```python
from build123d import *

# Parameters (mm, degrees)
F0_R     = 2.1
F1_DEPTH = 4


with BuildPart() as f1:
    # F0 (on Front) → F1 (new body)
    with BuildSketch(Plane.XZ):
        with BuildLine():
            ThreePointArc((-26.381971, 6.326054), (-23.972685, 2.787165), (-22.959026, -1.372268))
            ThreePointArc((-22.959026, -1.372268), (-21.551931, -8.032077), (-18.25719, -13.988388))
            ThreePointArc((-18.25719, -13.988388), (-14.253779, -16.291001), (-9.800476, -15.067308))
            Line((-9.800476, -15.067308), (-7.628003, -13.369986))
            ThreePointArc((-7.628003, -13.369986), (-5.887443, -12.424939), (-3.934034, -12.098051))
            Line((-3.934034, -12.098051), (3.934034, -12.098051))
            ThreePointArc((3.934034, -12.098051), (5.887443, -12.424939), (7.628003, -13.369986))
            Line((7.628003, -13.369986), (9.800476, -15.067308))
            ThreePointArc((9.800476, -15.067308), (14.253779, -16.291001), (18.25719, -13.988388))
            ThreePointArc((18.25719, -13.988388), (18.941172, 13.047299), (-6.562939, 22.043771))
            ThreePointArc((-6.562939, 22.043771), (-10.818219, 21.573689), (-14.967711, 22.627305))
            Line((-14.967711, 22.627305), (-29.819204, 29.402617))
            ThreePointArc((-29.819204, 29.402617), (-38.582061, 27.01545), (-37.828191, 17.964599))
            Line((-37.828191, 17.964599), (-26.381971, 6.326054))
        make_face()
        with BuildLine():
            ThreePointArc((11.244166, -10.473286), (9.304982, -9.523645), (7.182465, -9.127198))
            ThreePointArc((7.182465, -9.127198), (6.591412, -9.105339), (6, -9.098051))
            Line((6, -9.098051), (-6, -9.098051))
            ThreePointArc((-6, -9.098051), (-6.591412, -9.105339), (-7.182465, -9.127198))
            ThreePointArc((-7.182465, -9.127198), (-9.304982, -9.523645), (-11.244166, -10.473286))
            ThreePointArc((-11.244166, -10.473286), (-12.370984, -10.228297), (-12.082394, -9.11185))
            ThreePointArc((-12.082394, -9.11185), (-11.388234, -6.575), (-13.932291, -5.907735))
            ThreePointArc((-13.932291, -5.907735), (-15.091357, -5.492805), (-14.470173, -4.429916))
            ThreePointArc((-14.470173, -4.429916), (-12.950222, -2.283474), (-15.112635, -0.786331))
            ThreePointArc((-15.112635, -0.786331), (-16.059887, 0), (-15.112635, 0.786331))
            ThreePointArc((-15.112635, 0.786331), (-12.950222, 2.283474), (-14.470173, 4.429916))
            ThreePointArc((-14.470173, 4.429916), (-15.091357, 5.492805), (-13.932291, 5.907735))
            ThreePointArc((-13.932291, 5.907735), (-11.388234, 6.575), (-12.082394, 9.11185))
            ThreePointArc((-12.082394, 9.11185), (-12.302587, 10.323096), (-11.071506, 10.316579))
            ThreePointArc((-11.071506, 10.316579), (-8.452657, 10.073484), (-8.237301, 12.69476))
            ThreePointArc((-8.237301, 12.69476), (-8.029943, 13.90827), (-6.875335, 13.481092))
            ThreePointArc((-6.875335, 13.481092), (-4.497565, 12.356958), (-3.398667, 14.746495))
            ThreePointArc((-3.398667, 14.746495), (-2.78877, 15.815901), (-1.849896, 15.019585))
            ThreePointArc((-1.849896, 15.019585), (0, 13.15), (1.849896, 15.019585))
            ThreePointArc((1.849896, 15.019585), (2.78877, 15.815901), (3.398667, 14.746495))
            ThreePointArc((3.398667, 14.746495), (4.497565, 12.356958), (6.875335, 13.481092))
            ThreePointArc((6.875335, 13.481092), (8.029943, 13.90827), (8.237301, 12.69476))
            ThreePointArc((8.237301, 12.69476), (8.452657, 10.073484), (11.071506, 10.316579))
            ThreePointArc((11.071506, 10.316579), (12.302587, 10.323096), (12.082394, 9.11185))
            ThreePointArc((12.082394, 9.11185), (11.388234, 6.575), (13.932291, 5.907735))
            ThreePointArc((13.932291, 5.907735), (15.091357, 5.492805), (14.470173, 4.429916))
            ThreePointArc((14.470173, 4.429916), (12.950222, 2.283474), (15.112635, 0.786331))
            ThreePointArc((15.112635, 0.786331), (16.059887, 0), (15.112635, -0.786331))
            ThreePointArc((15.112635, -0.786331), (12.950222, -2.283474), (14.470173, -4.429916))
            ThreePointArc((14.470173, -4.429916), (15.091357, -5.492805), (13.932291, -5.907735))
            ThreePointArc((13.932291, -5.907735), (11.388234, -6.575), (12.082394, -9.11185))
            ThreePointArc((12.082394, -9.11185), (12.370984, -10.228297), (11.244166, -10.473286))
        make_face(mode=Mode.SUBTRACT)
        with Locations((-31.537354, 22.082693)):
            Circle(F0_R, mode=Mode.SUBTRACT)
    extrude(amount=F1_DEPTH)


solid = f1.part
```
Could you check a few things on this model? Use its own coordinates, in mm. A direction names the side the tool comes from. Round coordinates to 2 decimals unless told otherwise and drop trailing zeros. Loops run counter-clockwise (first coordinate to the right, second up) from the corner with the lowest first, then second, coordinate; pieces in that order, holes last. Notation, with made-up numbers: M 35,46.5 L 81,46.5 A16 cw 81,76.5 Z; hole C -20.5,86 d10. An arc over 180 degrees is marked long. Answer as CSV lines item,"result".
1) Imagine slicing it at A-A on x = 0. List the corners of the cut face in (y, z) for me.
From the geometry:
outline,"M -4,-12.1 L 0,-12.1 L 0,-9.1 L -4,-9.1 Z; M -4,13.15 L 0,13.15 L 0,23 L -4,23 Z"
2) Imagine slicing it at D-D on x = -35. List the corners of the cut face in (y, z) for me, and give its area (3 significant figures).
From the geometry:
outline,"M -4,15.09 L 0,15.09 L 0,29.68 L -4,29.68 Z"
area,"58.4 mm^2"
3) We'd pull the mould along Z, two halves only. Please class faces 4 (the cylindrical face through (12.944, -1.972, 2.324)), 5 (the cylindrical face through (-23.997, -1.972, 2.842)), 6 (the cylindrical face through (19.17, -1.97, 12.71)), 7 (the cylindrical face through (-4.54, -1.97, 12.34)): released by +Z, released by -Z, zero draft, split by the parting line, or undercut.
From the geometry:
face 4,"undercut"
face 5,"released by -Z"
face 6,"split by the parting line"
face 7,"undercut"
4) Imagine slicing it at B-B on z = -7.5. List the corners of the cut face in (x, y) for me, and give its area (3 significant figures).
From the geometry:
outline,"M -21.74,-4 L -11.14,-4 L -11.14,0 L -21.74,0 Z; M 11.14,-4 L 21.74,-4 L 21.74,0 L 11.14,0 Z"
area,"84.8 mm^2"
5) Imagine slicing it at C-C on y = -3.15. Count the separate pieces of the cut face and the enclosed holes in it, and give its area (3 significant figures).
From the geometry:
separate pieces,"1"
enclosed holes,"2"
area,"1,260 mm^2"
6) For pin 1 Ø1.5 at (x, y) = (-6.5, -3) entering from +Z; pin 2 Ø2 at (x, y) = (-1.5, -1) entering from -Z, each with a flat end and sliding along its axis, tell me the tip position at first contact or that it passes through.
From the geometry:
pin 1,"z = 22.27"
pin 2,"z = -12.1"
7) If I drill on probe 1 along Z at (x, y) = (-15, -2.5); probe 2 along X at (y, z) = (-0.65, -14); probe 3 along Z at (x, y) = (-13.5, -1.5), over which ranges is the centre line in solid material (lowest first)?
From the geometry:
probe 1,"-16.15 to -5.67, -4.77 to -0.77, 0.77 to 4.77, 5.67 to 22.64"
probe 2,"-18.25 to -8.43, 8.43 to 18.25"
probe 3,"-16.34 to -5.72, -3.95 to -1.26, 1.26 to 3.95, 5.72 to 22.07"
8) Which directions (+Z, -Z, +X, -X, +Y, -Y) give clear straight access to the entire face, cutting with the end or side of a thin tool? Please do faces 1 (the flat face through (-9, 0, 12)), 2 (the flat face through (8.7, -1.97, -14.21)), 3 (the cylindrical face through (9.33, -1.97, -9.53)).
From the geometry:
face 1,"+Z, -Z, +X, -X, +Y"
face 2,"-Z, +Y, -Y"
face 3,"+Y, -Y"
